from build123d import *

# Parameters (mm, degrees)
BOSS_EXTRUDE1_DEPTH = 3
FILLET1_R           = 0.2


with BuildPart() as part:
    # Sketch1 → Boss-Extrude1 (new body)
    with BuildSketch(Plane(origin=(0, 0, 0), x_dir=(1, 0, 0), z_dir=(0, 1, 0))):
        with BuildLine():
            Line((-2.5, 17), (-21, 17))
            ThreePointArc((-21, 17), (-22.414213562, 16.414213562), (-23, 15))
            Line((-23, 15), (-23, 3.660865618))
            ThreePointArc((-23, 3.660865618), (-22.636634177, 2.511331551), (-21.678571429, 1.779498876))
            ThreePointArc((-21.678571429, 1.779498876), (-10.791388434, 0.008370007), (0, 2.291697995))
            ThreePointArc((0, 2.291697995), (10.791388434, 0.008370007), (21.678571429, 1.779498876))
            ThreePointArc((21.678571429, 1.779498876), (22.636634177, 2.511331551), (23, 3.660865618))
            Line((23, 3.660865618), (23, 15))
            ThreePointArc((23, 15), (22.414213562, 16.414213562), (21, 17))
            Line((21, 17), (2.5, 17))
            Line((2.5, 17), (0, 14.5))
            Line((0, 14.5), (-2.5, 17))
        make_face()
        with BuildLine():
            Line((-10, 12), (-10, 4))
            ThreePointArc((-10, 4), (-11.5, 2.5), (-13, 4))
            Line((-13, 4), (-13, 12))
            ThreePointArc((-13, 12), (-11.5, 13.5), (-10, 12))
        make_face(mode=Mode.SUBTRACT)
        with BuildLine():
            Line((10, 12), (10, 4))
            ThreePointArc((10, 4), (11.5, 2.5), (13, 4))
            Line((13, 4), (13, 12))
            ThreePointArc((13, 12), (11.5, 13.5), (10, 12))
        make_face(mode=Mode.SUBTRACT)
    extrude(amount=BOSS_EXTRUDE1_DEPTH)

    # Fillet1
    fillet1_edges = [part.edges().sort_by_distance(p)[0] for p in [
        (-22.414213562, 3, -16.414213562),
        (1.25, 0, -15.75),
        (11.75, 0, -17),
        (22.414213562, 0, -16.414213562),
        (23, 0, -9.330432809),
        (22.636634177, 0, -2.511331551),
        (10.791388434, 0, -0.008370007),
        (-23, 3, -9.330432809),
        (-10.791388434, 0, -0.008370007),
        (-22.636634177, 0, -2.511331551),
        (-23, 0, -9.330432809),
        (-22.414213562, 0, -16.414213562),
        (-11.75, 0, -17),
        (-1.25, 0, -15.75),
        (-22.636634177, 3, -2.511331551),
        (-10.791388434, 3, -0.008370007),
        (0, 1.5, -14.5),
        (2.5, 1.5, -17),
        (0, 1.5, -2.291697995),
        (-2.5, 1.5, -17),
        (10.791388434, 3, -0.008370007),
        (22.636634177, 3, -2.511331551),
        (23, 3, -9.330432809),
        (22.414213562, 3, -16.414213562),
        (11.75, 3, -17),
        (1.25, 3, -15.75),
        (-1.25, 3, -15.75),
        (-11.75, 3, -17),
    ]]
    fillet(fillet1_edges, radius=FILLET1_R)


solid = part.part
Input: part model. Units: mm. Frame: model coordinates. A direction names the side the tool comes from. Coordinates: 2 decimals unless noted, no trailing zeros. Loops run counter-clockwise (first coordinate to the right, second up) from the corner with the lowest first, then second, coordinate; pieces in that order, holes last.
(1) Pull-direction query (X, two-part tool) for faces 5 (the face through (11.5, 1.5, -13.5)), 6 (the face through (0, 3, -9)), 7 (the face through (-22.4, 1.48, -16.43)); classes: released by +X, released by -X, zero draft, split by the parting line, or undercut.
(2) Section B-B on y = 2.15. Count the separate pieces of the cut face and the enclosed holes in it, then the cut area to 3 significant figures.
(3) Set-up query: faces 1 (the face through (-1.35, 2.94, -15.77)), 2 (the face through (-1.35, 0.06, -15.77)), 3 (the face through (-11.5, 1.5, -13.5)), 4 (the face through (-23, 1, -9)). Return all of +Z, -Z, +X, -X, +Y, -Y with unobstructed straight access to the full face (end or side cutting, diameter ignored); none if empty.
(4) Section A-A on z = -9. Return the cut outline in (x, y), then the cut area to 3 significant figures.
(5) Material intervals for probe 1 along X at (y, z) = (0.9, -8); probe 2 along X at (y, z) = (0.6, -12.5); probe 3 along Z at (x, y) = (13.5, 1.7), sorted ascending.
(6) First-contact query: pin 1 Ø1.5 at (x, z) = (11, -5) entering from -Y; pin 2 Ø1 at (x, y) = (-2, 2) entering from +Z. Flat tips, straight axial feed; report the tip coordinate or a pass-through.
Data:
1. face 5: undercut
1. face 6: zero draft
1. face 7: released by -X
2. separate pieces: 1
2. enclosed holes: 2
2. area: 677 mm2
3. face 1: -Z, +Y
3. face 2: -Z, -Y
3. face 3: +Y, -Y
3. face 4: +Z, -Z, -X, +Y, -Y
4. outline: (-23, 0.2) arc R0.2 ccw to (-22.8, 0) - (-13, 0) - (-13, 3) - (-22.8, 3) arc R0.2 ccw to (-23, 2.8) - close; (-10, 0) - (10, 0) - (10, 3) - (-10, 3) - close; (13, 0) - (22.8, 0) arc R0.2 ccw to (23, 0.2) - (23, 2.8) arc R0.2 ccw to (22.8, 3) - (13, 3) - close
4. area: 120 mm2
5. probe 1: x = -23 to -13, -10 to 10, 13 to 23
5. probe 2: x = -23 to -12.91, -10.09 to 10.09, 12.91 to 23
5. probe 3: z = -17 to -0.07
6. pin 1: passes through
6. pin 2: stops at z = -1.38
